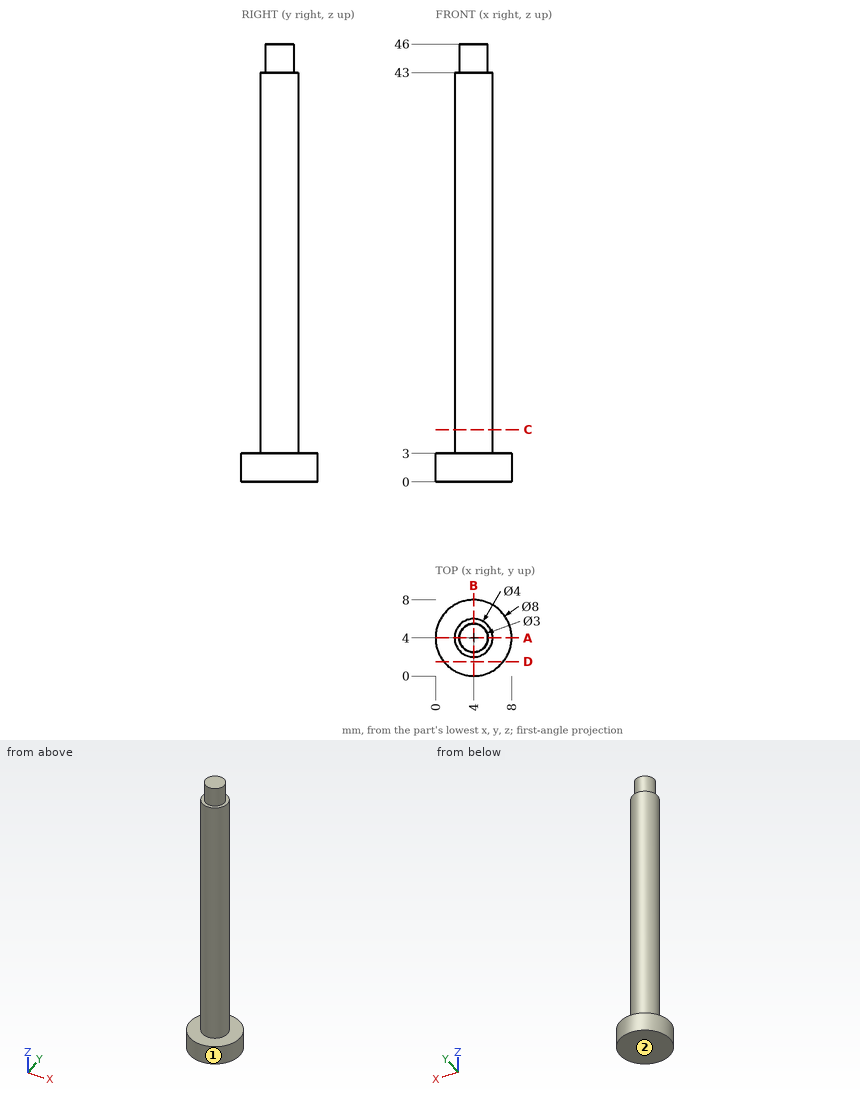
For this review, use the dimensioned drawing (mm, ordinates from the lowest corner) and the shaded views. Give positions to 0.01 mm unless a question says otherwise; leave off trailing zeros. Order: outer loops, then holes, each group sorted by start corner. A loop starts at its lowest first (then second) coordinate and runs counter-clockwise, first axis right, second up. Notation, with made-up numbers: (-2, -11.75) - (2, -11.75) arc R33 ccw to (2, 27.25) - close; hole circle Ø2 at (4.5, 1). An arc over 180 degrees is marked (long way). Use a Markdown table: item, result. Add a question column.
(1) Add section D-D on y = 1.5. Give the boundary of the cut face in (x, z).
(2) Wall thickness on probe 1 along Z at (x, y) = (2.25, 4); probe 2 along Z at (x, y) = (3, 6.75); probe 3 along Y at (x, z) = (5.25, 44): over which ranges is each line inside the solid? List them lowest first. Write a range as [from, to].
(3) Mouldability with a two-part tool opening along Z and no side actions: class the marked faces 1 and 2 as +Z half, -Z half, draft (parallel to the pull), parting line (faces both ways), or undercut.
(4) Add section C-C on z = 5.5. Give the boundary of the cut face in (x, y), then the cut area to 3 significant figures.
(5) Clearance check with flat-ended pins moving along their axes: P1, Ø1.5, axis at x = 5.5, z = 17.5, coming from the +Y side; P2, Ø3, axis at y = 3.5, z = 22, coming from the +X side; P3, Ø2, axis at x = 3, y = 6, coming from the -Z side; P4, Ø4, axis at x = 5.5, z = 8, coming from the -Y side. State where each tip first meets the part, or that it passes through.
(6) Add section A-A on y = 4. Give the boundary of the cut face in (x, z), then the cut area to 3 significant figures.
Report:
| question | item | result |
|---|---|---|
| 1 | outline | (0.88, 0) - (7.12, 0) - (7.12, 3) - (0.88, 3) - close |
| 2 | probe 1 | z = [0, 43] |
| 2 | probe 2 | z = [0, 3] |
| 2 | probe 3 | y = [3.17, 4.83] |
| 3 | face 1 | draft |
| 3 | face 2 | -Z half |
| 4 | outline | circle Ø4 at (4, 4) |
| 4 | area | 12.6 mm² |
| 5 | P1 | stops at y = 5.85 |
| 5 | P2 | stops at x = 6 |
| 5 | P3 | stops at z = 0 |
| 5 | P4 | stops at y = 2 |
| 6 | outline | (0, 0) - (8, 0) - (8, 3) - (6, 3) - (6, 43) - (5.5, 43) - (5.5, 46) - (2.5, 46) - (2.5, 43) - (2, 43) - (2, 3) - (0, 3) - close |
| 6 | area | 193 mm² |
